```python
from build123d import *

# Parameters (mm, degrees)
EXTRUDE_1_DEPTH              = 20
HOLE_WIZARD_5_8_1_AT_2_COUNT = 2
HOLE_WIZARD_5_8_1_AT_2_PITCH = 259.490550386
HOLE_WIZARD_5_8_1_AT_3_COUNT = 2
HOLE_WIZARD_5_8_1_AT_3_PITCH = 208.21625411
HOLE_WIZARD_5_8_1_AT_4_COUNT = 2
HOLE_WIZARD_5_8_1_AT_4_PITCH = 332.700096506
FILLET_1_R                   = 10


with BuildPart() as part:
    # 草图2 → 凸台-拉伸1 (new body)
    with BuildSketch(Plane(origin=(0, 0, 0), x_dir=(1, 0, 0), z_dir=(0, 1, 0))):
        with BuildLine():
            Line((-200, 160), (200, 160))
            ThreePointArc((200, 160), (207.071067812, 157.071067812), (210, 150))
            Line((210, 150), (210, 0))
            Line((210, 0), (210, -150))
            ThreePointArc((210, -150), (207.071067812, -157.071067812), (200, -160))
            Line((200, -160), (-200, -160))
            ThreePointArc((-200, -160), (-207.071067812, -157.071067812), (-210, -150))
            Line((-210, -150), (-210, 0))
            Line((-210, 0), (-210, 150))
            ThreePointArc((-210, 150), (-207.071067812, 157.071067812), (-200, 160))
        make_face()
        Polygon((-157.328690373, 132.321363833), (-171.715726709, 118.428445296), (-166.853205221, 113.392982578), (-152.466168885, 127.285901115), align=None, mode=Mode.SUBTRACT)
        Polygon((-171.715726709, -118.428445296), (-166.853205221, -113.392982578), (-152.466168885, -127.285901115), (-157.328690373, -132.321363833), align=None, mode=Mode.SUBTRACT)
        Polygon((157.328690373, -132.321363833), (171.715726709, -118.428445296), (166.853205221, -113.392982578), (152.466168885, -127.285901115), align=None, mode=Mode.SUBTRACT)
        Polygon((171.715726709, 118.428445296), (166.853205221, 113.392982578), (152.466168885, 127.285901115), (157.328690373, 132.321363833), align=None, mode=Mode.SUBTRACT)
    extrude(amount=EXTRUDE_1_DEPTH)

    # 草图16 → 5/8 六角头螺钉的柱形沉头孔1 (revolve, cut)
    with BuildSketch(Plane(origin=(-129.745275193, 0, 104.108127055), x_dir=(0, 0, -1), z_dir=(1, 0, 0))):
        Polygon((0, 0), (0, 20), (8.53313, 20), (8.53313, 11.2776), (17.4625, 11.2776), (17.4625, 0.532828266), (18.0975, 0), align=None)
    hole_wizard_5_8_1 = revolve(axis=Axis((-129.745275193, -6.35, 104.108127055), (0, 1, 0)), mode=Mode.SUBTRACT)

    # 5/8 六角头螺钉的柱形沉头孔1 at 2: 5/8 六角头螺钉的柱形沉头孔1 ×2
    with Locations(*[(i * HOLE_WIZARD_5_8_1_AT_2_PITCH, 0, 0) for i in range(1, HOLE_WIZARD_5_8_1_AT_2_COUNT)]):
        add(hole_wizard_5_8_1, mode=Mode.SUBTRACT)

    # 5/8 六角头螺钉的柱形沉头孔1 at 3: 5/8 六角头螺钉的柱形沉头孔1 ×2
    with Locations(*[(0, 0, -i * HOLE_WIZARD_5_8_1_AT_3_PITCH) for i in range(1, HOLE_WIZARD_5_8_1_AT_3_COUNT)]):
        add(hole_wizard_5_8_1, mode=Mode.SUBTRACT)

    # 5/8 六角头螺钉的柱形沉头孔1 at 4: 5/8 六角头螺钉的柱形沉头孔1 ×2
    with Locations(*[Vector(0.779953336687125, 0, -0.6258376727160331) * (i * HOLE_WIZARD_5_8_1_AT_4_PITCH) for i in range(1, HOLE_WIZARD_5_8_1_AT_4_COUNT)]):
        add(hole_wizard_5_8_1, mode=Mode.SUBTRACT)

    # 圆角1
    fillet_1_edges = [part.edges().sort_by_distance(p)[0] for p in [
        (-210, 0, 0),
        (0, 0, -160),
        (210, 0, 0),
        (0, 20, -160),
        (-210, 20, 0),
        (0, 20, 160),
        (210, 20, 0),
        (0, 0, 160),
        (207.071067812, 20, -157.071067812),
        (-207.071067812, 0, 157.071067812),
        (-207.071067812, 0, -157.071067812),
        (207.071067812, 20, 157.071067812),
    ]]
    fillet(fillet_1_edges, radius=FILLET_1_R - 0.0001)  # a hair under: the kernel refuses the full size


solid = part.part
```
Here's how the part is built. I have some questions about the finished solid (model axes, mm). A direction names the side the tool comes from. Round coordinates to 2 decimals unless told otherwise and drop trailing zeros. Use a Markdown table: item, result. Add a question column.
(1) Suppose I cut it at A-A, the plane y = 5.25. Count the separate pieces of the cut face and the enclosed holes in it, and give its area (3 significant figures).
(2) I need wall thicknesses on line 1 along X through (y, z) = (1.5, 101); line 2 along Z through (x, y) = (137, 15); line 3 along Z through (x, y) = (-131.5, 5). Which ranges of each line are inside material? Lowest first, please.
(3) For pin 1 Ø8 at (y, z) = (15.5, -107.5) entering from -X; pin 2 Ø17.5 at (x, z) = (125.5, -106) entering from -Y; pin 3 Ø1.5 at (x, y) = (4, 7) entering from -Z; pin 4 Ø10 at (x, y) = (32, 14) entering from +Z, each with a flat end and sliding along its axis, tell me the tip position at first contact or that it passes through.
(4) If we mould it in two halves opening along Z, with no side actions, what happens to faces 4 (the face through (2.8, 2.85, -156.99)), 5 (the face through (-207.15, 16.99, -2.1)), 6 (the face through (122, 11.278, -100))? For each: released by +Z, released by -Z, zero draft, split by the parting line, or undercut.
(5) For faces 1 (the face through (207.15, 16.99, 2.1)), 2 (the face through (159.76, 9.86, -120.24)), 3 (the face through (126, 11.278, 112)), which set-ups out of +Z, -Z, +X, -X, +Y, -Y let a thin tool reach every point of the face, with its end or its side?
Verdict:
| question | item | result |
|---|---|---|
| 1 | separate pieces | 1 |
| 1 | enclosed holes | 8 |
| 1 | area | 128,000 mm2 |
| 2 | line 1 | -205.27 to -146.93, -112.56 to 112.56, 146.93 to 205.27 |
| 2 | line 2 | -158.66 to -108.6, -99.62 to 99.62, 108.6 to 158.66 |
| 2 | line 3 | -158.66 to -121.48, -86.73 to 86.73, 121.48 to 158.66 |
| 3 | pin 1 | x = -209.89 |
| 3 | pin 2 | y = 11.28 |
| 3 | pin 3 | z = -159.74 |
| 3 | pin 4 | z = 160 |
| 4 | face 4 | released by -Z |
| 4 | face 5 | zero draft |
| 4 | face 6 | undercut |
| 5 | face 1 | +Z, -Z, +X, +Y |
| 5 | face 2 | +Y, -Y |
| 5 | face 3 | -Y |
